```python
from build123d import *

# Parameters (mm, degrees)
SKETCH1_R           = 30
BOSS_EXTRUDE1_DEPTH = 17.5
SKETCH2_W           = 33
SKETCH2_H           = 33
BOSS_EXTRUDE2_DEPTH = 120
SKETCH3_R           = 15
BOSS_EXTRUDE3_DEPTH = 20
CUT_EXTRUDE1_START  = -40
CUT_EXTRUDE1_DEPTH  = 194.968340902
CIRPATTERN1_COUNT   = 4
HOLE1_D             = 30


with BuildPart() as part:
    # Sketch1 → Boss-Extrude1 (new, symmetric)
    with BuildSketch(Plane(origin=(0, 0, 0), x_dir=(1, 0, 0), z_dir=(0, 1, 0))):
        with Locations(Location((0, 0, 0), (0, 0, 270))):
            Circle(SKETCH1_R)
    extrude(amount=BOSS_EXTRUDE1_DEPTH, both=True)

    # Sketch2 → Boss-Extrude2 (add)
    with BuildSketch(Plane.XY):
        Rectangle(SKETCH2_W, SKETCH2_H)
    extrude(amount=BOSS_EXTRUDE2_DEPTH)

    # Sketch3 → Boss-Extrude3 (add)
    with BuildSketch(Plane.XY.offset(120)):
        Circle(SKETCH3_R)
    extrude(amount=BOSS_EXTRUDE3_DEPTH)

    # Sketch4 → Cut-Extrude1 (cut)
    with BuildSketch(Plane.XY.offset(120).offset(CUT_EXTRUDE1_START)):
        with BuildLine():
            Line((16.5, 11.5), (16.5, 16.5))
            Line((16.5, 16.5), (11.5, 16.5))
            ThreePointArc((11.5, 16.5), (12.964466094, 12.964466094), (16.5, 11.5))
        make_face()
    cut_extrude1 = extrude(amount=CUT_EXTRUDE1_DEPTH, mode=Mode.SUBTRACT)

    # CirPattern1: Cut-Extrude1 ×4 about axis
    cirpattern1_axis = Axis((0, 0, 0), (0, 0, 1))
    for i in range(1, CIRPATTERN1_COUNT):
        add(cut_extrude1.rotate(cirpattern1_axis, i * 360 / CIRPATTERN1_COUNT), mode=Mode.SUBTRACT)

    # Hole1 (through all)
    with Locations(Plane(origin=(0, 17.5, 0), x_dir=(1, 0, 0), z_dir=(0, 1, 0))):
        with Locations((0, 0)):
            Hole(HOLE1_D / 2)


solid = part.part
```
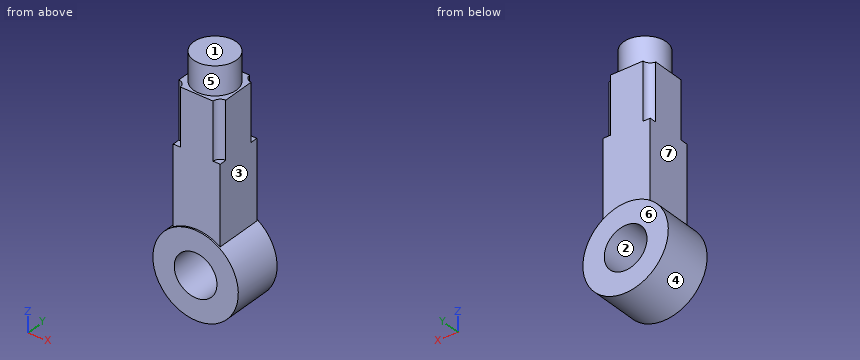
CAD build for the part. Positions are in the model's coordinates, mm. Face numbers are marked on the shaded views. A direction names the side the tool comes from. Coordinates: 2 decimals unless noted, no trailing zeros. Order: outer loops, then holes, each group sorted by start corner. A loop starts at its lowest first (then second) coordinate and runs counter-clockwise, first axis right, second up. Notation, with made-up numbers: M -9,40.25 L 20,40.25 A26 ccw 20,73.25 Z; hole C 74,10.5 d9. An arc over 180 degrees is marked long. Answer as CSV lines item,"result".
1) Drill centre lines: L1, parallel to X at y = 1, z = 101; L2, parallel to X at y = 4.5, z = 7; L3, parallel to X at y = 5, z = 4. Where is each one in solid material? Low to high. Write a range as from..to.
Verdict:
L1,"-16.5..16.5"
L2,"-29.17..-13.27, 13.27..29.17"
L3,"-29.73..-14.46, 14.46..29.73"
2) Cut at D-D (z = 70). List the corners of the cut face in (x, y), then the cut area to 3 significant figures.
Verdict:
outline,"M -16.5,-16.5 L 16.5,-16.5 L 16.5,16.5 L -16.5,16.5 Z"
area,"1,090 mm2"
3) Flat gauge pins, fed straight in: P1, Ø8, axis at y = 9.5, z = 118.5, coming from the +X side; P2, Ø2, axis at x = 7, y = -8.5, coming from the -Z side; P3, Ø10, axis at y = 1, z = 21, coming from the -X side. Where does each tip first touch, or does it go through?
Verdict:
P1,"x = 16.5"
P2,"z = -29.39"
P3,"x = -25.38"
4) Cut at B-B (y = 0). List the corners of the cut face in (x, z).
Verdict:
outline,"M -16.5,25.05 A30 ccw long 16.5,25.05 L 16.5,120 L 15,120 L 15,140 L -15,140 L -15,120 L -16.5,120 Z; hole C 0,0 d30"
5) Cut at C-C (z = 0). List the corners of the cut face in (x, y).
Verdict:
outline,"M -30,-17.5 L -15,-17.5 L -15,17.5 L -30,17.5 Z; M 15,-17.5 L 30,-17.5 L 30,17.5 L 15,17.5 Z"
6) Mould opens along Z. For the marked faces 1, 2, 3 and 4 say: released by +Z, released by -Z, zero draft, split by the parting line, or undercut.
Verdict:
face 1,"released by +Z"
face 2,"undercut"
face 3,"zero draft"
face 4,"split by the parting line"
7) Cut at A-A (x = 0). List the corners of the cut face in (y, z), then the cut area to 3 significant figures.
Verdict:
outline,"M -17.5,-30 L 17.5,-30 L 17.5,-15 L -17.5,-15 Z; M -17.5,15 L 17.5,15 L 17.5,30 L 16.5,30 L 16.5,120 L 15,120 L 15,140 L -15,140 L -15,120 L -16.5,120 L -16.5,30 L -17.5,30 Z"
area,"4,620 mm2"
8) 3-axis set-ups, long thin cutter, end or side, ignore diameter. For the marked faces 5, 6 and 7: which of +Z, -Z, +X, -X, +Y, -Y reach the whole face in a straight line?
Verdict:
face 5,"+Z"
face 6,"+Z, -Z, +X, -X, +Y"
face 7,"+Z, -X, +Y, -Y"
